Here's the drawing with two shaded views (mm, measured from the low corner). I have some questions. A direction names the side the tool comes from. Coordinates: 2 decimals unless noted, no trailing zeros. Loops run counter-clockwise (first coordinate to the right, second up) from the corner with the lowest first, then second, coordinate; pieces in that order, holes last.
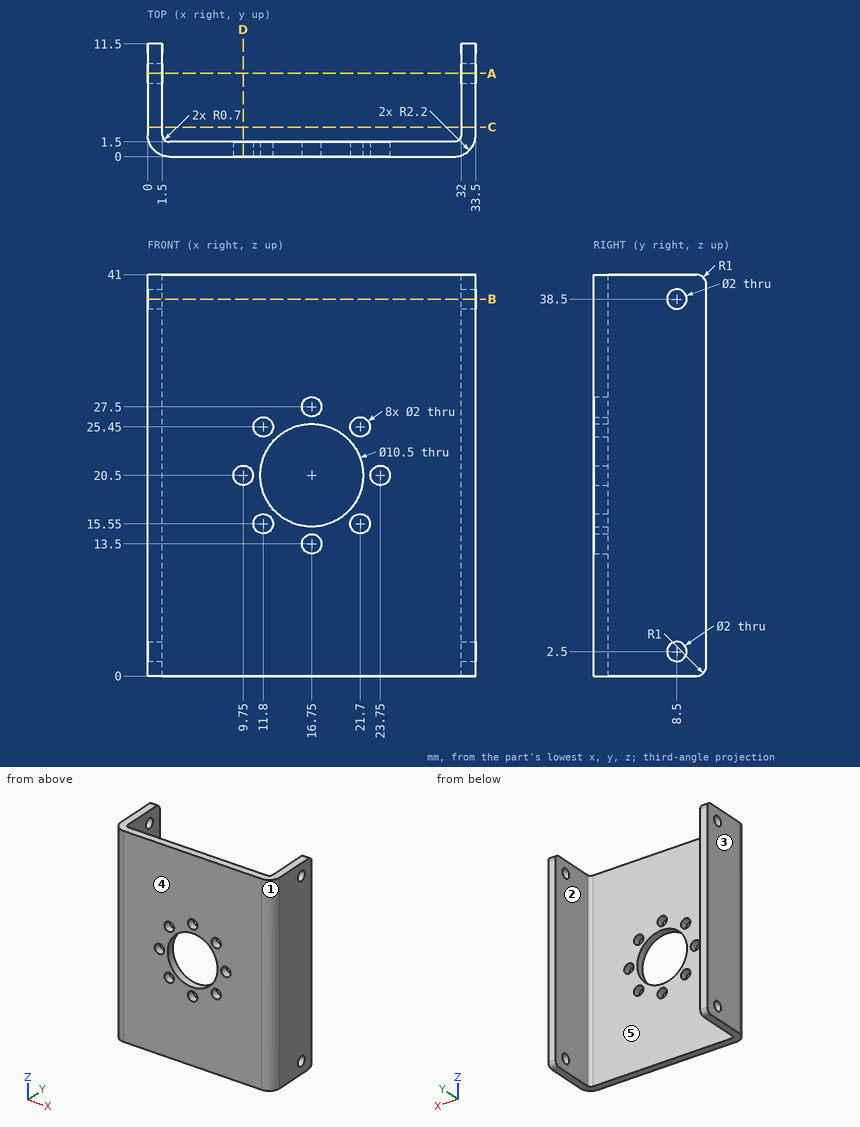
(1) I want a section at B-B on z = 38.5. Write out the boundary of the cut face in (x, y).
Check values:
outline: (0, 2.2) arc R2.2 ccw to (2.2, 0) - (31.3, 0) arc R2.2 ccw to (33.5, 2.2) - (33.5, 7.5) - (32, 7.5) - (32, 2.2) arc R0.7 cw to (31.3, 1.5) - (2.2, 1.5) arc R0.7 cw to (1.5, 2.2) - (1.5, 7.5) - (0, 7.5) - close; (0, 9.5) - (1.5, 9.5) - (1.5, 11.5) - (0, 11.5) - close; (32, 9.5) - (33.5, 9.5) - (33.5, 11.5) - (32, 11.5) - close
(2) If we mould it in two halves opening along X, with no side actions, what happens to the marked faces 3, 4 and 5? For each: released by +X, released by -X, zero draft, split by the parting line, or undercut.
Check values:
face 3: released by -X
face 4: zero draft
face 5: undercut
(3) I want a section at D-D on x = 9.75. Write out the boundary of the cut face in (y, z).
Check values:
outline: (0, 0) - (1.5, 0) - (1.5, 19.5) - (0, 19.5) - close; (0, 21.5) - (1.5, 21.5) - (1.5, 41) - (0, 41) - close
(4) Which directions (+Z, -Z, +X, -X, +Y, -Y) give clear straight access to the entire face, cutting with the end or side of a thin tool? Please do the marked faces 1 and 2.
Check values:
face 1: +Z, -Z, +X, -Y
face 2: +Z, -Z, +Y
(5) I want a section at A-A on y = 8.5. Write out the boundary of the cut face in (x, z).
Check values:
outline: (0, 0) - (1.5, 0) - (1.5, 1.5) - (0, 1.5) - close; (0, 3.5) - (1.5, 3.5) - (1.5, 37.5) - (0, 37.5) - close; (0, 39.5) - (1.5, 39.5) - (1.5, 41) - (0, 41) - close; (32, 0) - (33.5, 0) - (33.5, 1.5) - (32, 1.5) - close; (32, 3.5) - (33.5, 3.5) - (33.5, 37.5) - (32, 37.5) - close; (32, 39.5) - (33.5, 39.5) - (33.5, 41) - (32, 41) - close
(6) I'm going to push a flat-ended pin straight in: pin 1 (12 mm diameter, centred on x = 16.5, z = 20.5, fed in from +Y). Where does the tip first touch, or does it pass through?
Check values:
pin 1: stops at y = 1.5
(7) I want a section at C-C on y = 3. Write out the boundary of the cut face in (x, z), then the cut area to 3 significant figures.
Check values:
outline: (0, 0) - (1.5, 0) - (1.5, 41) - (0, 41) - close; (32, 0) - (33.5, 0) - (33.5, 41) - (32, 41) - close
area: 123 mm2
(8) If I drill on probe 1 along Z at (x, y) = (0.3, 8.5); probe 2 along X at (y, z) = (9.25, 31.5); probe 3 along Z at (x, y) = (12.5, 0.75) (1 decimal), over which ranges is the centre line in solid material (lowest first)?
Check values:
probe 1: z = 0 to 1.5, 3.5 to 37.5, 39.5 to 41
probe 2: x = 0 to 1.5, 32 to 33.5
probe 3: z = 0 to 14.8, 16.3 to 17.4, 23.6 to 24.7, 26.2 to 41
